```python
from build123d import *

# Parameters (mm, degrees)
SKETCH1_R             = 7.9375
SKETCH1_R_2           = 11.1125
BOSS_EXTRUDE1_DEPTH   = 12.7
F_8_CLEARANCE_HOLE1_D = 4.4958
SKETCH5_R             = 18.415
CUT_EXTRUDE1_DEPTH    = 218.842023092
SKETCH7_R             = 9.525
CUT_EXTRUDE2_DEPTH    = 218.842023092
CUT_EXTRUDE3_DEPTH    = 218.842023092
BOSS_EXTRUDE2_DEPTH   = 12.7
CUT_EXTRUDE4_DEPTH    = 218.842023092
SKETCH11_W            = 12.7
SKETCH11_H            = 178.054
CUT_EXTRUDE5_DEPTH    = 3.175
BOSS_EXTRUDE3_DEPTH   = 6.35
CUT_EXTRUDE6_DEPTH    = 253.498549798
FILLET1_R             = 12.7
SKETCH16_W            = 6.35
SKETCH16_H            = 25.4
BOSS_EXTRUDE4_DEPTH   = 6.35
CUT_EXTRUDE7_DEPTH    = 253.258895086
FILLET2_R             = 9.525
FILLET3_R             = 25.4


with BuildPart() as part:
    # Sketch1 → Boss-Extrude1 (new body)
    with BuildSketch(Plane(origin=(0, 0, 0), x_dir=(0, 0, -1), z_dir=(1, 0, 0))):
        with BuildLine():
            Line((93.345, 0), (55.245, 50.8))
            Line((55.245, 50.8), (-160.655, 50.8))
            ThreePointArc((-160.655, 50.8), (-211.455, 0), (-160.655, -50.8))
            Line((-160.655, -50.8), (55.245, -50.8))
            Line((55.245, -50.8), (93.345, 0))
        make_face()
        with Locations((-88.9, 0)):
            Circle(SKETCH1_R, mode=Mode.SUBTRACT)
        with Locations((-38.1, 0)):
            Circle(SKETCH1_R, mode=Mode.SUBTRACT)
        with Locations((-160.655, 0)):
            Circle(SKETCH1_R_2, mode=Mode.SUBTRACT)
        Circle(SKETCH1_R, mode=Mode.SUBTRACT)
    extrude(amount=BOSS_EXTRUDE1_DEPTH)

    # #8 Clearance Hole1 (through all)
    with Locations(Plane.ZY):
        with Locations((-17.691104559, 17.691104559), (17.691104559, 17.691104559), (17.691104559, -17.691104559), (-17.691104559, -17.691104559)):
            Hole(F_8_CLEARANCE_HOLE1_D / 2)

    # Sketch5 → Cut-Extrude1 (cut, through all)
    with BuildSketch(Plane.ZY):
        Circle(SKETCH5_R)
    extrude(amount=-CUT_EXTRUDE1_DEPTH, mode=Mode.SUBTRACT)

    # Sketch7 → Cut-Extrude2 (cut, through all)
    with BuildSketch(Plane.ZY):
        with Locations((-55.245, 0)):
            Circle(SKETCH7_R)
    extrude(amount=-CUT_EXTRUDE2_DEPTH, mode=Mode.SUBTRACT)

    # Sketch8 → Cut-Extrude3 (cut, through all)
    with BuildSketch(Plane(origin=(12.7, 0, 0), x_dir=(0, 0, -1), z_dir=(1, 0, 0))):
        Polygon((-160.655, 50.8), (-211.455, 25.4), (-211.455, -25.4), (-160.655, -50.8), (-233.239745749, -50.8), (-233.239745749, 50.8), align=None)
    extrude(amount=-CUT_EXTRUDE3_DEPTH, mode=Mode.SUBTRACT)

    # Sketch9 → Boss-Extrude2 (add)
    with BuildSketch(Plane(origin=(12.7, 0, 0), x_dir=(0, 0, -1), z_dir=(1, 0, 0))):
        Polygon((-160.655, 50.8), (-211.455, 25.4), (-211.455, 0), (-211.455, -25.4), (-160.655, -50.8), (-160.655, -40.64), (-202.749323348, 0), (-160.655, 40.64), align=None)
    extrude(amount=-BOSS_EXTRUDE2_DEPTH)

    # Sketch10 → Cut-Extrude4 (cut, through all)
    with BuildSketch(Plane.ZY):
        Polygon((-79.0575, -19.05), (-79.0575, 19.05), (-93.345, 0), align=None)
    extrude(amount=-CUT_EXTRUDE4_DEPTH, mode=Mode.SUBTRACT)

    # Sketch11 → Cut-Extrude5 (cut)
    with BuildSketch(Plane(origin=(0, 50.8, 0), x_dir=(1, 0, 0), z_dir=(0, 1, 0))):
        with Locations((6.35, -52.705)):
            Rectangle(SKETCH11_W, SKETCH11_H)
    cut_extrude5 = extrude(amount=-CUT_EXTRUDE5_DEPTH, mode=Mode.SUBTRACT)

    # Mirror1: Cut-Extrude5 across plane
    add(cut_extrude5.mirror(Plane.ZX), mode=Mode.SUBTRACT)

    # Sketch13 → Cut-Extrude6 (cut, through all)
    with BuildSketch(Plane(origin=(12.7, 0, 0), x_dir=(0, 0, -1), z_dir=(1, 0, 0))):
        Polygon((-161.254612663, -53.34), (-139.192, -53.34), (-139.192, -50.165), (33.782, -50.165), (33.782, -53.34), (56.515, -53.34), (81.5975, -19.896666667), (81.5975, 19.896666667), (56.515, 53.34), (33.782, 53.34), (33.782, 50.165), (-139.192, 50.165), (-139.192, 53.34), (-161.254612663, 53.34), (-213.995, 26.969806331), (-213.995, -26.969806331), align=None)
    extrude(amount=-CUT_EXTRUDE6_DEPTH, mode=Mode.SUBTRACT)


with BuildPart() as body_2:
    # Sketch12 → Boss-Extrude3 (new body)
    with BuildSketch(Plane(origin=(12.7, 0, 0), x_dir=(0, 0, -1), z_dir=(1, 0, 0))):
        with BuildLine():
            ThreePointArc((-211.89681554, -56.397839854), (-236.855, 0), (-211.89681554, 56.397839854))
            Line((-211.89681554, 56.397839854), (-243.205, 43.989212666))
            Line((-243.205, 43.989212666), (-243.205, -43.989212666))
            Line((-243.205, -43.989212666), (-211.89681554, -56.397839854))
        make_face()
        with BuildLine():
            Line((-217.805, 29.324515829), (-162.154031657, 57.15))
            Line((-162.154031657, 57.15), (-166.916531657, 66.675))
            Line((-166.916531657, 66.675), (-185.966531657, 66.675))
            Line((-185.966531657, 66.675), (-211.89681554, 56.397839854))
            ThreePointArc((-211.89681554, 56.397839854), (-236.855, 0), (-211.89681554, -56.397839854))
            Line((-211.89681554, -56.397839854), (-185.966531657, -66.675))
            Line((-185.966531657, -66.675), (-166.916531657, -66.675))
            Line((-166.916531657, -66.675), (-162.154031657, -57.15))
            Line((-162.154031657, -57.15), (-217.805, -29.324515829))
            Line((-217.805, -29.324515829), (-217.805, 29.324515829))
        make_face()
    extrude(amount=-BOSS_EXTRUDE3_DEPTH)

    # Fillet1
    fillet1_edges = [body_2.edges().sort_by_distance(p)[0] for p in [
        (9.525, -43.989212666, 243.205),
        (9.525, 43.989212666, 243.205),
        (9.525, 66.675, 185.966531657),
        (9.525, 66.675, 166.916531657),
        (9.525, -66.675, 166.916531657),
        (9.525, -66.675, 185.966531657),
    ]]
    fillet(fillet1_edges, radius=FILLET1_R)

    # Sketch16 → Boss-Extrude4 (add)
    with BuildSketch(Plane(origin=(12.7, 0, 0), x_dir=(0, 0, -1), z_dir=(1, 0, 0))):
        with Locations((-214.63, 0)):
            Rectangle(SKETCH16_W, SKETCH16_H)
        Polygon((-178.620290503, -48.916870577), (-175.780484171, -43.237257914), (-198.498934823, -31.878032589), (-201.338741154, -37.557645251), align=None)
        Polygon((-201.338741154, 37.557645251), (-198.498934823, 31.878032589), (-175.780484171, 43.237257914), (-178.620290503, 48.916870577), align=None)
    extrude(amount=-BOSS_EXTRUDE4_DEPTH)

    # Sketch17 → Cut-Extrude7 (cut, through all)
    with BuildSketch(Plane(origin=(12.7, 0, 0), x_dir=(0, 0, -1), z_dir=(1, 0, 0))):
        with BuildLine():
            Line((-174.765563314, 66.675), (-183.541544079, 66.675))
            ThreePointArc((-183.541544079, 66.675), (-185.923497883, 66.44962609), (-188.220911491, 65.781503319))
            Line((-188.220911491, 65.781503319), (-235.184367412, 47.168095163))
            ThreePointArc((-235.184367412, 47.168095163), (-241.010188388, 42.498188858), (-243.205, 35.361591844))
            Line((-243.205, 35.361591844), (-243.205, -35.361591844))
            ThreePointArc((-243.205, -35.361591844), (-241.010188388, -42.498188858), (-235.184367412, -47.168095163))
            Line((-235.184367412, -47.168095163), (-188.220911491, -65.781503319))
            ThreePointArc((-188.220911491, -65.781503319), (-185.923497883, -66.44962609), (-183.541544079, -66.675))
            Line((-183.541544079, -66.675), (-174.765563314, -66.675))
            ThreePointArc((-174.765563314, -66.675), (-171.322248813, -66.199303058), (-168.136883002, -64.80784807))
            Line((-168.136883002, -64.80784807), (-197.079031657, -50.336773743))
            Line((-197.079031657, -50.336773743), (-227.33, -35.211289571))
            Line((-227.33, -35.211289571), (-227.33, -3.175))
            Line((-227.33, -3.175), (-227.33, 3.175))
            Line((-227.33, 3.175), (-227.33, 35.211289571))
            Line((-227.33, 35.211289571), (-197.079031657, 50.336773743))
            Line((-197.079031657, 50.336773743), (-168.136883002, 64.80784807))
            ThreePointArc((-168.136883002, 64.80784807), (-171.322248813, 66.199303058), (-174.765563314, 66.675))
        make_face()
    extrude(amount=-CUT_EXTRUDE7_DEPTH, mode=Mode.SUBTRACT)

    # Fillet2
    # the kernel refuses this fillet: 9.525 mm, written as the material it takes off along each edge
    with BuildSketch(Plane(origin=(36.994694288, -64.80784807, 168.136883002), x_dir=(0, 0.4472135954999565, 0.8944271909999166), z_dir=(-1, 0, 0))) as fillet2_piece_1:
        with BuildLine():
            CenterArc((7.598468847, 9.525), FILLET2_R, 180, 90)
            Line((-1.926531153, 9.525), (-2.879031153, 9.525))
            ThreePointArc((-2.879031153, 9.525), (-2.879031153, 6.724757914), (-0.808010164, -0.504356844))
            Line((-0.808010164, -0.504356844), (0, -0.9525))
            Line((0, -0.9525), (7.598468847, -0.9525))
            Line((7.598468847, -0.9525), (7.598468847, 0))
        make_face()
    extrude(amount=54.939388575, mode=Mode.SUBTRACT)
    with BuildSketch(Plane(origin=(36.994694288, 64.80784807, 168.136883002), x_dir=(0, -0.447213595499958, 0.894427190999916), z_dir=(-1, 0, 0))) as fillet2_piece_2:
        with BuildLine():
            CenterArc((7.598468847, -9.525), FILLET2_R, 90, 90)
            Line((-1.926531153, -9.525), (-2.879031153, -9.525))
            ThreePointArc((-2.879031153, -9.525), (-2.879031153, -6.724757914), (-0.808010164, 0.504356844))
            Line((-0.808010164, 0.504356844), (0, 0.9525))
            Line((0, 0.9525), (7.598468847, 0.9525))
            Line((7.598468847, 0.9525), (7.598468847, 0))
        make_face()
    extrude(amount=54.939388575, mode=Mode.SUBTRACT)

    # Fillet3
    fillet3_edges = [body_2.edges().sort_by_distance(p)[0] for p in [
        (9.525, 35.211289571, 227.33),
        (9.525, -35.211289571, 227.33),
    ]]
    fillet(fillet3_edges, radius=FILLET3_R)


solid = body_2.part
```
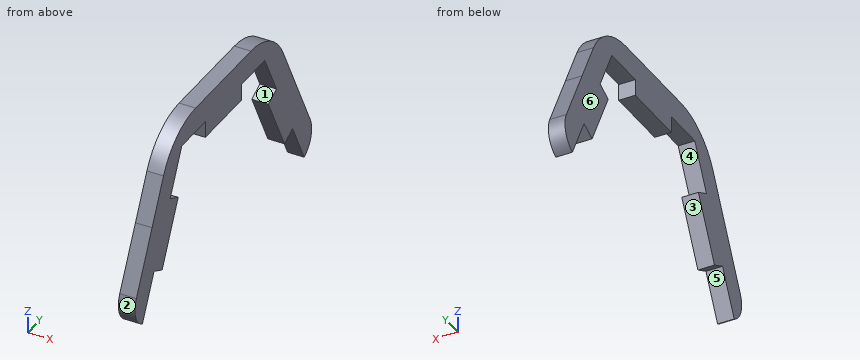
Source: CAD feature listing. Evaluate the final solid. Frame: model axes, mm. Face numbers are marked on the shaded views. A direction names the side the tool comes from. Give positions to 0.01 mm unless a question says otherwise; leave off trailing zeros. Write each loop counter-clockwise with the first axis right and the second up, starting at its lowest first coordinate (ties: lowest second). Pieces come first, ordered by that corner, then holes. Notation, with made-up numbers: (-32.75, 13.25) - (-16.75, 13.25) arc R37 cw to (-16.75, 49.25) - close; hole circle Ø11 at (68.25, 11). An arc over 180 degrees is marked (long way). One line per item, written item: value. Start each with the question number.
Q1. Draft query along Z for the marked faces 4, 5 and 6. Return one class per face: +Z half, -Z half, draft (parallel to the pull), parting line (faces both ways), or undercut.
Q2. Section query D-D, the plane z = 203. Return the cut outline in (x, y).
Q3. Section query C-C, the plane y = 8.5. Return the cut outline in (x, z) (3 decimals).
Q4. First-contact query: pin 1 Ø3 at (x, z) = (9.5, 216) entering from -Y; pin 2 Ø3 at (x, z) = (9, 180) entering from -Y; pin 3 Ø1.5 at (x, y) = (9.5, 29.5) entering from +Z. Flat tips, straight axial feed; report the tip coordinate or a pass-through.
Q5. Section query A-A, the plane x = 7.5. Return the cut outline in (y, z) (3 decimals).
Q6. Section query B-B, the plane z = 182. Return the cut outline in (x, y), then the cut area to 3 significant figures.
Q7. Material intervals for probe 1 along Y at (x, z) = (9, 215); probe 2 along Z at (x, y) = (11, 11.5) (3 decimals); probe 3 along Z at (x, y) = (10.75, -35) (3 decimals), sorted ascending. Write a range as from..to.
Q8. Set-up query: the marked faces 1, 2 and 3. Return all of +Z, -Z, +X, -X, +Y, -Y with unobstructed straight access to the full face (end or side cutting, diameter ignored); none if empty.
Answer:
1. face 4: undercut
1. face 5: -Z half
1. face 6: draft
2. outline: (6.35, -47.38) - (12.7, -47.38) - (12.7, -36.73) - (6.35, -36.73) - close; (6.35, 36.73) - (12.7, 36.73) - (12.7, 47.38) - (6.35, 47.38) - close
3. outline: (6.35, 211.455) - (12.7, 211.455) - (12.7, 227.33) - (6.35, 227.33) - close
4. pin 1: stops at y = -41.58
4. pin 2: stops at y = -59.63
4. pin 3: stops at z = 225.59
5. outline: (-61.41, 174.933) arc R9.525 ccw to (-57.15, 162.154) - (-48.917, 178.62) - (-43.237, 175.78) - (-31.878, 198.499) - (-37.558, 201.339) - (-29.325, 217.805) - (-12.7, 217.805) - (-12.7, 211.455) - (12.7, 211.455) - (12.7, 217.805) - (29.325, 217.805) - (37.558, 201.339) - (31.878, 198.499) - (43.237, 175.78) - (48.917, 178.62) - (57.15, 162.154) arc R9.525 ccw to (61.41, 174.933) - (42.232, 213.289) arc R25.4 ccw to (19.513, 227.33) - (-19.513, 227.33) arc R25.4 ccw to (-42.232, 213.289) - close
6. outline: (6.35, -57.88) - (12.7, -57.88) - (12.7, -40.13) - (6.35, -40.13) - close; (6.35, 40.13) - (12.7, 40.13) - (12.7, 57.88) - (6.35, 57.88) - close
6. area: 225 mm2
7. probe 1: y = -41.29..-30.73, -12.7..12.7, 30.73..41.29
7. probe 2: z = 211.455..227.33
7. probe 3: z = 192.255..200.06, 206.454..222.063
8. face 1: +X, -X
8. face 2: +X, -X, -Y
8. face 3: -Z, +X, -X
